```python
from build123d import *

# Parameters (mm, degrees)
SKETCH1_R           = 10
BOSS_EXTRUDE1_DEPTH = 65
SKETCH2_R           = 1.65
CUT_EXTRUDE1_DEPTH  = 15
CHAMFER1_SIZE       = 0.5
SKETCH3_R           = 5
CUT_EXTRUDE2_DEPTH  = 15
CHAMFER2_SIZE       = 0.5
CHAMFER3_SIZE       = 0.5
SKETCH4_W           = 24.548279796
SKETCH4_H           = 20
CUT_EXTRUDE3_DEPTH  = 13


with BuildPart() as part:
    # Sketch1 → Boss-Extrude1 (new body)
    with BuildSketch(Plane.XY):
        Circle(SKETCH1_R)
    extrude(amount=BOSS_EXTRUDE1_DEPTH)

    # Sketch2 → Cut-Extrude1 (cut)
    with BuildSketch(Plane.XY.offset(65)):
        Circle(SKETCH2_R)
    extrude(amount=-CUT_EXTRUDE1_DEPTH, mode=Mode.SUBTRACT)

    # Chamfer1
    chamfer1_edges = [part.edges().sort_by_distance(p)[0] for p in [
        (-1.65, 0, 65),
    ]]
    chamfer(chamfer1_edges, length=CHAMFER1_SIZE)

    # Sketch3 → Cut-Extrude2 (cut)
    with BuildSketch(Plane(origin=(0, 0, 0), x_dir=(-1, 0, 0), z_dir=(0, 0, -1))):
        Circle(SKETCH3_R)
    extrude(amount=-CUT_EXTRUDE2_DEPTH, mode=Mode.SUBTRACT)

    # Chamfer2
    chamfer2_edges = [part.edges().sort_by_distance(p)[0] for p in [
        (5, 0, 0),
    ]]
    chamfer(chamfer2_edges, length=CHAMFER2_SIZE)

    # Chamfer3
    chamfer3_edges = [part.edges().sort_by_distance(p)[0] for p in [
        (-10, 0, 0),
    ]]
    chamfer(chamfer3_edges, length=CHAMFER3_SIZE)

    # Sketch4 → Cut-Extrude3 (cut)
    with BuildSketch(Plane(origin=(0, 0, 0), x_dir=(1, 0, 0), z_dir=(0, 1, 0))):
        with Locations((0.075917463, -30)):
            Rectangle(SKETCH4_W, SKETCH4_H)
    extrude(amount=-CUT_EXTRUDE3_DEPTH, mode=Mode.SUBTRACT)


solid = part.part
```
Here's how the part is built. I have some questions about the finished solid (model axes, mm). A direction names the side the tool comes from. Coordinates: 2 decimals unless noted, no trailing zeros. Loops run counter-clockwise (first coordinate to the right, second up) from the corner with the lowest first, then second, coordinate; pieces in that order, holes last. Notation, with made-up numbers: (58.25, 79) - (78.25, 79) arc R13 ccw to (78.25, 101) - close; hole circle Ø3 at (-39, 45). An arc over 180 degrees is marked (long way). Return JSON: item names as keys, results as strings. Group by question number.
Item 1: Will these pins go through, and if not, where does the flat tip stop? P1, Ø6, axis at x = 0, y = 0, coming from the -Z side; P2, Ø5, axis at x = 2, z = 55.5, coming from the +Y side; P3, Ø6, axis at y = 4.5, z = 33, coming from the +X side; P4, Ø1.6, axis at x = 0, y = 0.5, coming from the +Z side.
Item 2: On a 3-axis mill with a long thin cutter (end or side, diameter ignored), from which of +Z, -Z, +X, -X, +Y, -Y can I reach the whole of each face in a straight line? I mean faces 1 (the face through (0, 0, 15)), 2 (the face through (0, 0, 50)), 3 (the face through (0, 0, 30)). Say none if no direction works.
Item 3: I need wall thicknesses on line 1 (Y direction, x = 0, z = 7.5); line 2 (Z direction, x = 8, y = -3.75); line 3 (Z direction, x = 2.75, y = 1.25). Which ranges of each line are inside material? Lowest first, please. Write a range as from..to.
Item 4: If we section it at A-A on x = 0: Write out the boundary of the cut face in (y, z), and give its area (3 significant figures).
Item 5: If we section it at C-C on z = 42: Write out the boundary of the cut face in (x, y).
Item 6: If we section it at D-D on z = 10: Write out the boundary of the cut face in (x, y), and give its area (3 significant figures).
Item 7: If we section it at B-B on z = 56: Write out the boundary of the cut face in (x, y), and give its area (3 significant figures).
Item 8: We'd pull the mould along Y, two halves only. Please class faces 4 (the face through (1.08, -4.88, 7.65)), 5 (the face through (4, -4, 0)), 6 (the face through (-1.302, 9.915, 32.298)): +Y half, -Y half, draft (parallel to the pull), parting line (faces both ways), or undercut.
Calculated:
{
 "1": {"P1": "stops at z = 15", "P2": "stops at y = 10", "P3": "stops at x = 9.89", "P4": "stops at z = 50"},
 "2": {"face 1": "-Z", "face 2": "+Z", "face 3": "+X, -X, -Y"},
 "3": {"line 1": "y = -10..-5, 5..10", "line 2": "z = 0..20, 40..65", "line 3": "z = 15..65"},
 "4": {"outline": "(-10, 0.5) - (-9.5, 0) - (-5.5, 0) - (-5, 0.5) - (-5, 15) - (5, 15) - (5, 0.5) - (5.5, 0) - (9.5, 0) - (10, 0.5) - (10, 65) - (2.15, 65) - (1.65, 64.5) - (1.65, 50) - (-1.65, 50) - (-1.65, 64.5) - (-2.15, 65) - (-10, 65) - (-10, 40) - (0, 40) - (0, 20) - (-10, 20) - close", "area": "900 mm^2"},
 "5": {"outline": "circle Ø20 at (0, 0)"},
 "6": {"outline": "circle Ø20 at (0, 0); hole circle Ø10 at (0, 0)", "area": "236 mm^2"},
 "7": {"outline": "circle Ø20 at (0, 0); hole circle Ø3.3 at (0, 0)", "area": "306 mm^2"},
 "8": {"face 4": "undercut", "face 5": "draft", "face 6": "parting line"}
}
